The model under review builds one solid part; all positions refer to its coordinate system, in mm. Coordinates: 2 decimals unless noted, no trailing zeros. Loops run counter-clockwise (first coordinate to the right, second up) from the corner with the lowest first, then second, coordinate; pieces in that order, holes last. Notation, with made-up numbers: M -23.75,-40 L 19.25,-40 A34 cw 19.25,-3 Z; hole C 13.25,39 d9. An arc over 180 degrees is marked long. One line per item, written item: value.
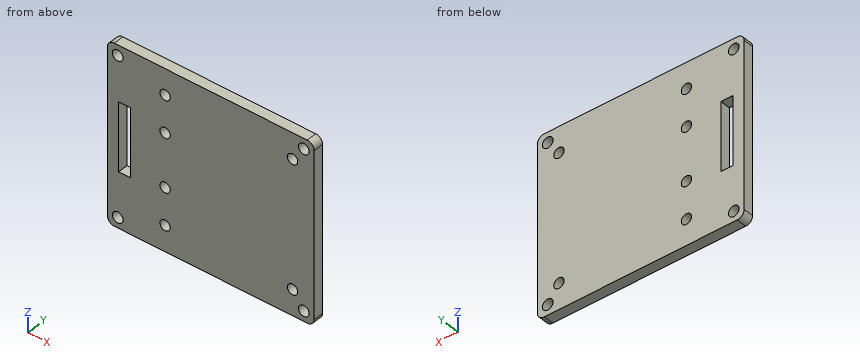
```python
from build123d import *

# Parameters (mm, degrees)
SKETCH1_W           = 60
SKETCH1_H           = 52
SKETCH1_R           = 1.5
SKETCH1_R_2         = 1.55
SKETCH1_W_2         = 3.5
SKETCH1_H_2         = 19.9
BOSS_EXTRUDE1_DEPTH = 3
FILLET1_R           = 2


with BuildPart() as part:
    # Sketch1 → Boss-Extrude1 (new body)
    with BuildSketch(Plane(origin=(0, 0, 0), x_dir=(1, 0, 0), z_dir=(0, 1, 0))):
        with Locations((-5.25, 0)):
            Rectangle(SKETCH1_W, SKETCH1_H)
        with Locations(Location((-18.5, -18.5, 0), (0, 0, 270))):
            Circle(SKETCH1_R, mode=Mode.SUBTRACT)
        with Locations(Location((-18.5, 18.5, 0), (0, 0, 270))):
            Circle(SKETCH1_R, mode=Mode.SUBTRACT)
        with Locations(Location((18.5, 18.5, 0), (0, 0, 270))):
            Circle(SKETCH1_R, mode=Mode.SUBTRACT)
        with Locations(Location((18.5, -18.5, 0), (0, 0, 270))):
            Circle(SKETCH1_R, mode=Mode.SUBTRACT)
        with Locations(Location((-18.5, -7.75, 0), (0, 0, 270))):
            Circle(SKETCH1_R, mode=Mode.SUBTRACT)
        with Locations(Location((-18.5, 7.75, 0), (0, 0, 270))):
            Circle(SKETCH1_R, mode=Mode.SUBTRACT)
        with Locations(Location((-32.25, 23, 0), (0, 0, 270))):
            Circle(SKETCH1_R_2, mode=Mode.SUBTRACT)
        with Locations(Location((21.75, 23, 0), (0, 0, 270))):
            Circle(SKETCH1_R_2, mode=Mode.SUBTRACT)
        with Locations(Location((21.75, -23, 0), (0, 0, 270))):
            Circle(SKETCH1_R_2, mode=Mode.SUBTRACT)
        with Locations(Location((-32.25, -23, 0), (0, 0, 270))):
            Circle(SKETCH1_R_2, mode=Mode.SUBTRACT)
        with Locations((-30.25, 0)):
            Rectangle(SKETCH1_W_2, SKETCH1_H_2, mode=Mode.SUBTRACT)
    extrude(amount=BOSS_EXTRUDE1_DEPTH)

    # Fillet1
    fillet1_edges = [part.edges().sort_by_distance(p)[0] for p in [
        (-35.25, 1.5, -26),
        (24.75, 1.5, -26),
        (24.75, 1.5, 26),
        (-35.25, 1.5, 26),
    ]]
    fillet(fillet1_edges, radius=FILLET1_R)


solid = part.part
```
(1) To check wall thickness, follow L1, parallel to X at y = 1.35, z = 18.5; L2, parallel to X at y = 2.2, z = 23; L3, parallel to X at y = 1.45, z = -1. State the ranges of each line that lie inside material, in increasing order. Write a range as [from, to].
Checks:
L1: [-35.25, -20], [-17, 17], [20, 24.75]
L2: [-35.25, -33.8], [-30.7, 20.2], [23.3, 24.75]
L3: [-35.25, -32], [-28.5, 24.75]
(2) Add section B-B on z = -7.75. State the section outline as (x, y) points.
Checks:
outline: M -35.25,0 L -32,0 L -32,3 L -35.25,3 Z; M -28.5,0 L -20,0 L -20,3 L -28.5,3 Z; M -17,0 L 24.75,0 L 24.75,3 L -17,3 Z
(3) Add section A-A on x = 18.5. State the section outline as (y, z) points.
Checks:
outline: M 0,-26 L 3,-26 L 3,-20 L 0,-20 Z; M 0,-17 L 3,-17 L 3,17 L 0,17 Z; M 0,20 L 3,20 L 3,26 L 0,26 Z
(4) Insertion check: pin 1 Ø1.8 at (x, z) = (-18.5, 18.5) entering from -Y. The pin has a flat end and moves straight along its axis. Give the tip position at first contact, or say it passes through.
Checks:
pin 1: through
(5) Add section C-C on y = 0.5. State how many separate pieces and enclosed holes the cut face has, then the cut area to 3 significant figures.
Checks:
separate pieces: 1
enclosed holes: 11
area: 2,970 mm^2
